Input: part model. Units: mm. Frame: model coordinates. Round coordinates to 2 decimals unless told otherwise and drop trailing zeros. Write each loop counter-clockwise with the first axis right and the second up, starting at its lowest first coordinate (ties: lowest second). Pieces come first, ordered by that corner, then holes. Notation, with made-up numbers: (66.25, 89.5) -> (106.25, 89.5) arc R18 cw to (106.25, 120.5) -> close; hole circle Ø9 at (-32, -31). An arc over 180 degrees is marked (long way). Use CSV: the item, a comma, the result in double quotes.
```python
from build123d import *

# Parameters (mm, degrees)
SKETCH1_R           = 3.4
BOSS_EXTRUDE1_DEPTH = 4.5
SKETCH2_R           = 1
CUT_EXTRUDE1_DEPTH  = 10
FILLET1_R           = 1


with BuildPart() as part:
    # Sketch1 → Boss-Extrude1 (new body)
    with BuildSketch(Plane.XY):
        Circle(SKETCH1_R)
    extrude(amount=BOSS_EXTRUDE1_DEPTH)

    # Sketch2 → Cut-Extrude1 (cut)
    with BuildSketch(Plane(origin=(4, 0, 0), x_dir=(0, 0, -1), z_dir=(1, 0, 0))):
        with Locations(Location((-2, 0, 0), (0, 0, 180))):
            Circle(SKETCH2_R)
    extrude(amount=-CUT_EXTRUDE1_DEPTH, mode=Mode.SUBTRACT)

    # Fillet1
    fillet1_edges = [part.edges().sort_by_distance(p)[0] for p in [
        (-3.4, 0, 0),
    ]]
    fillet(fillet1_edges, radius=FILLET1_R - 0.0001)  # a hair under: the kernel refuses the full size


solid = part.part
```
Item 1: Section query C-C on z = 1.4. Return the cut outline in (x, y).
Worked answers:
outline,"(-3.3, -0.8) arc R3.4 ccw to (3.3, -0.8) -> close; (-3.3, 0.8) -> (3.3, 0.8) arc R3.4 ccw to start"
Item 2: Line query: line 1 (Y direction, x = 0, z = 2); line 2 (Y direction, x = 1.25, z = 2); line 3 (Z direction, x = -1.75, y = 0.5). Output: solid intervals per line, ascending.
Worked answers:
line 1,"y = -3.4 to -1, 1 to 3.4"
line 2,"y = -3.16 to -1, 1 to 3.16"
line 3,"z = 0 to 1.13, 2.87 to 4.5"
Item 3: Section query B-B on x = 0. Return the cut outline in (y, z), plus the area to 3 significant figures.
Worked answers:
outline,"(-3.4, 1) arc R1 ccw to (-2.4, 0) -> (2.4, 0) arc R1 ccw to (3.4, 1) -> (3.4, 4.5) -> (-3.4, 4.5) -> close; hole circle Ø2 at (0, 2)"
area,"27.0 mm²"
Item 4: Section query D-D on z = 3.75. Return the cut outline in (x, y), plus the area to 3 significant figures.
Worked answers:
outline,"circle Ø6.8 at (0, 0)"
area,"36.3 mm²"
Item 5: Pull-direction query (Y, two-part tool) for faces 1 (the face through (3.14, -1.3, 2.73)), 2 (the face through (0, 0, 4.5)), 3 (the face through (0, 0.6, 1.2)); classes: +Y half, -Y half, draft (parallel to the pull), parting line (faces both ways), or undercut.
Worked answers:
face 1,"parting line"
face 2,"draft"
face 3,"undercut"
